Work out the finished part from the listing and answer in its coordinate system (mm). Coordinates: 2 decimals unless noted, no trailing zeros. Order: outer loops, then holes, each group sorted by start corner. A loop starts at its lowest first (then second) coordinate and runs counter-clockwise, first axis right, second up. Notation, with made-up numbers: M -37.75,22 L 17.25,22 A11 cw 17.25,42 Z; hole C -29.75,85 d7. An arc over 180 degrees is marked long. Use a Markdown table: item, result. Add a question column.
from build123d import *

# Parameters (mm, degrees)
SKETCH_1_R          = 22.5
EXTRUDE_1_DEPTH     = 1
SKETCH_2_R          = 40
EXTRUDE_2_DEPTH     = 1
SKETCH_3_R          = 7.5
CUT_EXTRUDE_1_DEPTH = 500
SKETCH_5_R          = 22.5
SKETCH_5_R_2        = 15
CUT_EXTRUDE_3_DEPTH = 1


with BuildPart() as part:
    # 草图1 → 凸台-拉伸1 (new body)
    with BuildSketch(Plane(origin=(0, 0, 0), x_dir=(1, 0, 0), z_dir=(0, 1, 0))):
        with Locations(Location((0, 0, 0), (0, 0, 270))):
            Circle(SKETCH_1_R)
    extrude(amount=EXTRUDE_1_DEPTH)

    # 草图2 → 凸台-拉伸2 (add)
    with BuildSketch(Plane(origin=(0, 1, 0), x_dir=(1, 0, 0), z_dir=(0, 1, 0))):
        with Locations(Location((0, 0, 0), (0, 0, 270))):
            Circle(SKETCH_2_R)
    extrude(amount=EXTRUDE_2_DEPTH)

    # 草图3 → 切除-拉伸1 (cut)
    with BuildSketch(Plane(origin=(0, 2, 0), x_dir=(1, 0, 0), z_dir=(0, 1, 0))):
        with Locations(Location((0, 0, 0), (0, 0, 270))):
            Circle(SKETCH_3_R)
    extrude(amount=-CUT_EXTRUDE_1_DEPTH, mode=Mode.SUBTRACT)

    # 草图5 → 切除-拉伸3 (cut)
    with BuildSketch(Plane.XZ):
        Circle(SKETCH_5_R)
        with Locations(Location((0, 0, 0), (0, 0, 270))):
            Circle(SKETCH_5_R_2, mode=Mode.SUBTRACT)
    extrude(amount=-CUT_EXTRUDE_3_DEPTH, mode=Mode.SUBTRACT)


solid = part.part
(1) Straight lines are drawn through the part: line 1 (X direction, y = 1.25, z = 0); line 2 (X direction, y = 0.7, z = 0); line 3 (Y direction, x = 25, z = -1). For each, find the intervals that lie inside material, in ascending order.
(2) The mould has two halves that part along Z. Classify faces 1 (the cylindrical face through (0.33, 1.014, -7.493)), 2 (the flat face through (1, 1, 17)), 3 (the cylindrical face through (0.66, 0.493, 14.985)): pulls with the +Z half, pulls with the -Z half, needs draft (parallel to the pull), parting line crosses it, or undercut.
(3) A cutting plane is placed at D-D on x = -32. Write down the section's boundary in (y, z), plus the area to 3 significant figures.
(4) A cutting plane is placed at C-C on y = 1.3. Write down the section's boundary in (x, z), plus the area to 3 significant figures.
(5) A cutting plane is placed at A-A on z = 0. Write down the section's boundary in (x, y).
(6) Given P1, Ø1, axis at x = -22.5, z = 0.5, coming from the -Y side, flat-ended and moving along its own axis, determine where the tip first touches the part or whether it passes through.
(7) A cutting plane is placed at B-B on x = 0. Write down the section's boundary in (y, z).
From the geometry:
| question | item | result |
|---|---|---|
| 1 | line 1 | x = -40 to -7.5, 7.5 to 40 |
| 1 | line 2 | x = -15 to -7.5, 7.5 to 15 |
| 1 | line 3 | y = 1 to 2 |
| 2 | face 1 | undercut |
| 2 | face 2 | needs draft |
| 2 | face 3 | parting line crosses it |
| 3 | outline | M 1,-24 L 2,-24 L 2,24 L 1,24 Z |
| 3 | area | 48.0 mm2 |
| 4 | outline | C 0,0 d80; hole C 0,0 d15 |
| 4 | area | 4,850 mm2 |
| 5 | outline | M -40,1 L -15,1 L -15,0 L -7.5,0 L -7.5,2 L -40,2 Z; M 7.5,0 L 15,0 L 15,1 L 40,1 L 40,2 L 7.5,2 Z |
| 6 | P1 | stops at y = 1 |
| 7 | outline | M 0,-15 L 1,-15 L 1,-40 L 2,-40 L 2,-7.5 L 0,-7.5 Z; M 0,7.5 L 2,7.5 L 2,40 L 1,40 L 1,15 L 0,15 Z |
